Autodesk Inventor part; units mm, degrees
ref_plane "YZ Plane" through (0, 0, 0) normal (1, 0, 0) x (0, 1, 0)
ref_plane "XZ Plane" through (0, 0, 0) normal (0, 1, 0) x (-1, 0, 0)
ref_plane "XY Plane" through (0, 0, 0) normal (0, 0, 1) x (1, 0, 0)
sketch "Boceto1" plane through (0, 0, 0) normal (0, 1, 0) x (-1, 0, 0)
  circle A0 centre (0, 0) radius 62
  circle A1 centre (0, 0) radius 72
  circle A2 centre (0, 0) radius 52
  dimension "d5" = 124
  dimension "d6" = 144
  dimension "d7" = 104
extrude "Extrusión1" add sketch "Boceto1" along normal blind 100 contours A1
sketch "Boceto5" plane through (0, 0, 0) normal (0, -1, 0) x (1, 0, 0)
  circle A0 centre (0, 0) radius 52
  circle A1 centre (0, 0) radius 62
  dimension "d11" = 104
  dimension "d12" = 124
extrude "Extrusión2" add sketch "Boceto5" against normal blind 95
sketch "Boceto6" plane through (0, 0, 0) normal (0, -1, 0) x (1, 0, 0)
  circle A0 centre (0, 0) radius 52
  circle A1 centre (0, 0) radius 62
  dimension "d15" = 104
  dimension "d16" = 124
extrude "Extrusión3" cut sketch "Boceto6" against normal blind 80
sketch "Boceto7" plane through (0, 0, 0) normal (0, -1, 0) x (1, 0, 0)
  circle A0 centre (0, 0) radius 82
  circle A1 centre (0, 0) radius 72
  dimension "d19" = 164
  dimension "d20" = 144
extrude "Extrusión4" add sketch "Boceto7" against normal blind 15
fillet "Empalme1" radius 15 1 edges at (-82, 15, 0)
sketch "Boceto8" plane through (0, 0, 0) normal (0, -1, 0) x (1, 0, 0)
  arc A0 (43.8491, 43.8321) -> (16.8777, 59.6586) centre (0, 0) ccw
  line L0 (43.8491, 43.8321) -> (50.9216, 50.9018)
  line L1 (16.8777, 59.6586) -> (19.5999, 69.2809)
  line L2 (19.5999, 69.2809) -> (21.3442, 75.4464)
  line L3 (21.3442, 75.4464) -> (55.4532, 55.4317)
  line L4 (55.4532, 55.4317) -> (50.9216, 50.9018)
  dimension "d25" = 124
extrude "Extrusión5" cut sketch "Boceto8" against normal blind 30
sketch "Boceto9" plane through (0, 95, 0) normal (0, 1, 0) x (1, 0, 0)
  line L0 (51.775, -4.7614) -> (51.775, 6.1116)
  line L1 (5.2843, 55.289) -> (-4.7157, 55.289)
  line L2 (5.2843, 55.289) -> (5.2843, -56.0708)
  line L3 (5.2843, -56.0708) -> (-4.7157, -56.0708)
  line L4 (-4.7157, -56.0708) -> (-4.7157, 55.289)
  line L5 (5.2843, 55.289) -> (-4.7157, 55.289)
  line L6 (5.2843, 55.289) -> (5.2843, -56.0708)
  line L7 (5.2843, -56.0708) -> (-4.7157, -56.0708)
  line L8 (-4.7157, -56.0708) -> (-4.7157, 55.289)
  line L9 (-56.1571, 4.9777) -> (-56.1571, -5.0223)
  line L10 (-56.1571, 4.9777) -> (55.2027, 4.9777)
  line L11 (55.2027, 4.9777) -> (55.2027, -5.0223)
  line L12 (55.2027, -5.0223) -> (-56.1571, -5.0223)
extrude "Extrusión6" cut sketch "Boceto9" against normal blind 10
sketch "Boceto10" plane through (0, 85, 0) normal (0, 1, 0) x (1, 0, 0)
  line L0 (-51.7569, -5.0223) -> (-56.1571, -5.0223)
  line L1 (55.2027, -5.0223) -> (51.7569, -5.0223)
  line L2 (-56.1571, -5.0223) -> (55.2027, -5.0223)
  line L3 (55.2027, -5.0223) -> (55.2027, 4.9777)
  line L4 (-56.1571, 4.9777) -> (-51.7612, 4.9777)
  line L5 (55.2027, 4.9777) -> (-56.1571, 4.9777)
  line L6 (-56.1571, -5.0223) -> (-56.1571, 4.9777)
  line L7 (-56.1571, 4.9777) -> (-56.1571, -5.0223)
  line L8 (-4.7157, -56.0708) -> (-4.7157, -51.7857)
  line L9 (5.2843, -56.0708) -> (-4.7157, -56.0708)
  line L10 (-4.7157, -56.0708) -> (5.2843, -56.0708)
  line L11 (5.2843, 55.289) -> (5.2843, 51.7308)
  line L12 (5.2843, -56.0708) -> (5.2843, 55.289)
  line L13 (-4.7157, 55.289) -> (5.2843, 55.289)
  line L14 (5.2843, 55.289) -> (-4.7157, 55.289)
  line L15 (-4.7157, 55.289) -> (-4.7157, -56.0708)
  point P0 (0, 0)
extrude "Extrusión7" add sketch "Boceto10" along normal blind 8
sketch "Boceto11" plane through (0, 85, 0) normal (0, -1, 0) x (1, 0, 0)
  line L0 (0, 0) -> (0, -9.6645)
properties part number "BaseRod_Pepu"
Can you work these out from the model? Positions are in its coordinate system, mm. A direction names the side the tool comes from. Coordinates: 2 decimals unless noted, no trailing zeros. Order: outer loops, then holes, each group sorted by start corner. A loop starts at its lowest first (then second) coordinate and runs counter-clockwise, first axis right, second up.
1. If we section it at B-B (z = 0): Please give me the cut outline in (x, y), then the cut area to 3 significant figures.
2. If we section it at A-A (x = 0): Please give me the cut outline in (y, z).
3. I'm going to push flat-ended pins straight in: pin 1 (9 mm diameter, centred on y = 90, z = -28, fed in from +X); pin 2 (9 mm diameter, centred on x = -30.5, y = 87.5, fed in from +Z); pin 3 (4 mm diameter, centred on y = 87.5, z = 34, fed in from +X). Where does each tip first touch, or does it pass through?
4. Thinking about a two-plate mould opening in X: for faces 1 (the face through (18, 0, -60)), 2 (the face through (9.373, 56.905, -71.387)), 3 (the face through (0, 85, 0)), which applies, +X half, -X half, draft (parallel to the pull), parting line (faces both ways), or undercut?
5. If we section it at C-C (y = 47.5): Please give me the cut outline in (x, z).
6. If we section it at D-D (z = 29.5): Give the number of separate pieces and of enclosed holes in the cut face, then the cut area to 3 significant figures.
7. For faces 4 (the face through (-14.07, 95, -50.23)), 5 (the face through (5.284, 89, 29)), 6 (the face through (-49.2, 39.44, -37.73)), which set-ups out of +Z, -Z, +X, -X, +Y, -Y let a thin tool reach every point of the face, with its end or its side?
8. I need wall thicknesses on line 1 (X direction, y = 96, z = 0); line 2 (Z direction, x = -32, y = 9). Which ranges of each line are inside material? Lowest first, please.
Entries:
1. outline: (-82, 0) - (-62, 0) - (-62, 80) - (-52, 80) - (-52, 85) - (52, 85) - (52, 80) - (62, 80) - (62, 0) - (82, 0) - (82, 0.86) arc R15 ccw to (72, 15) - (72, 100) - (62, 100) - (62, 95) - (55.2, 95) - (55.2, 93) - (-56.16, 93) - (-56.16, 95) - (-62, 95) - (-62, 100) - (-72, 100) - (-72, 15) arc R15 ccw to (-82, 0.86) - close
1. area: 3,340 mm2
2. outline: (0, -82) - (0.86, -82) arc R15 ccw to (15, -72) - (100, -72) - (100, -62) - (95, -62) - (95, -55.29) - (93, -55.29) - (93, 56.07) - (95, 56.07) - (95, 62) - (100, 62) - (100, 72) - (15, 72) arc R15 ccw to (0.86, 82) - (0, 82) - (0, 62) - (80, 62) - (80, 52) - (85, 52) - (85, -52) - (80, -52) - (80, -62) - (0, -62) - close
3. pin 1: stops at x = 68.06
3. pin 2: stops at z = 67.14
3. pin 3: stops at x = 64.5
4. face 1: draft
4. face 2: parting line
4. face 3: undercut
5. outline: circle Ø144 at (0, 0); hole circle Ø124 at (0, 0)
6. separate pieces: 3
6. enclosed holes: 0
6. area: 2,900 mm2
7. face 4: +Y
7. face 5: +Y, -Y
7. face 6: -Y
8. line 1: x = -72 to -62, 62 to 72
8. line 2: z = -72.88 to -53.1, 53.1 to 72.88
